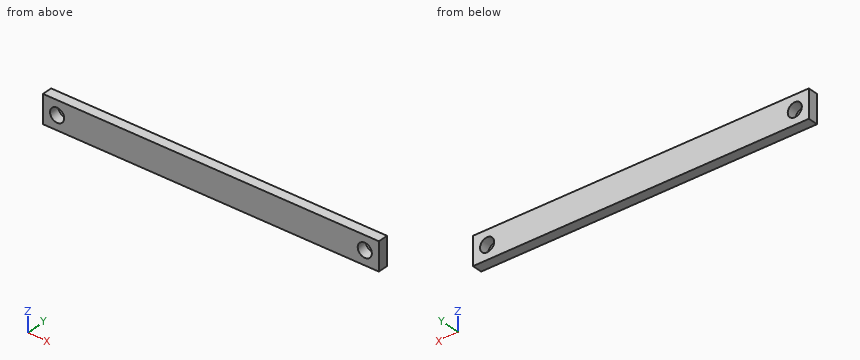
from build123d import *

# Parameters (mm, degrees)
ESQUISSE1_W             = 520
ESQUISSE1_H             = 42
BOSS_EXTRU_1_DEPTH      = 15
ESQUISSE2_R             = 10.5
ENL_V_MAT_EXTRU_1_DEPTH = 15
ESQUISSE3_W             = 10
ESQUISSE3_H             = 42
ENL_V_MAT_EXTRU_2_DEPTH = 262.277630118


with BuildPart() as part:
    # Esquisse1 → Boss.-Extru.1 (new body)
    with BuildSketch(Plane(origin=(0, 0, 0), x_dir=(1, 0, 0), z_dir=(0, 1, 0))):
        Rectangle(ESQUISSE1_W, ESQUISSE1_H)
    extrude(amount=BOSS_EXTRU_1_DEPTH)

    # Esquisse2 → Enlèv. mat.-Extru.1 (cut)
    with BuildSketch(Plane(origin=(0, 15, 0), x_dir=(1, 0, 0), z_dir=(0, 1, 0))):
        with Locations(Location((-229, 0, 0), (0, 0, 270))):
            Circle(ESQUISSE2_R)
        with Locations(Location((229, 0, 0), (0, 0, 270))):
            Circle(ESQUISSE2_R)
    extrude(amount=-ENL_V_MAT_EXTRU_1_DEPTH, mode=Mode.SUBTRACT)

    # Esquisse3 → Enlèv. mat.-Extru.2 (cut, through all)
    with BuildSketch(Plane(origin=(0, 15, 0), x_dir=(1, 0, 0), z_dir=(0, 1, 0))):
        with Locations((-255, 0)):
            Rectangle(ESQUISSE3_W, ESQUISSE3_H)
        with Locations((255, 0)):
            Rectangle(ESQUISSE3_W, ESQUISSE3_H)
    extrude(amount=-ENL_V_MAT_EXTRU_2_DEPTH, mode=Mode.SUBTRACT)


solid = part.part
Verification items for the finished model (mm, model axes). Coordinates: 2 decimals unless noted, no trailing zeros. Order: outer loops, then holes, each group sorted by start corner. A loop starts at its lowest first (then second) coordinate and runs counter-clockwise, first axis right, second up.
Item 1: Section check C-C, the plane y = 5. Enter the section's corners in (x, z), then the cut area to 3 significant figures.
Filled in:
outline: (-250, -21) - (250, -21) - (250, 21) - (-250, 21) - close; hole circle Ø21 at (-229, 0); hole circle Ø21 at (229, 0)
area: 20,300 mm2
Item 2: Material ranges on L1, parallel to X at y = 6.75, z = 0; L2, parallel to X at y = 2.25, z = -6.5; L3, parallel to Z at x = 220, y = 1.25, recorded low to high.
Filled in:
L1: x = -250 to -239.5, -218.5 to 218.5, 239.5 to 250
L2: x = -250 to -237.25, -220.75 to 220.75, 237.25 to 250
L3: z = -21 to -5.41, 5.41 to 21
Item 3: Section check A-A, the plane x = 229. Enter the section's corners in (y, z).
Filled in:
outline: (0, -21) - (15, -21) - (15, -10.5) - (0, -10.5) - close; (0, 10.5) - (15, 10.5) - (15, 21) - (0, 21) - close
Item 4: Section check B-B, the plane z = 0. Enter the section's corners in (x, y), then the cut area to 3 significant figures.
Filled in:
outline: (-250, 0) - (-239.5, 0) - (-239.5, 15) - (-250, 15) - close; (-218.5, 0) - (218.5, 0) - (218.5, 15) - (-218.5, 15) - close; (239.5, 0) - (250, 0) - (250, 15) - (239.5, 15) - close
area: 6,870 mm2
